```python
from build123d import *

# Parameters (mm, degrees)
SKETCH1_W           = 1025.461280364
SKETCH1_H           = 299.73488768
BOSS_EXTRUDE1_DEPTH = 19
SKETCH2_W           = 967.6
SKETCH2_H           = 175.74
CUT_EXTRUDE1_DEPTH  = 19
SKETCH3_R           = 7
CUT_EXTRUDE2_DEPTH  = 19
SKETCH5_W           = 19
SKETCH5_H           = 80
CUT_EXTRUDE3_DEPTH  = 19
SKETCH6_W           = 19
SKETCH6_H           = 80
CUT_EXTRUDE4_DEPTH  = 19


with BuildPart() as part:
    # Sketch1 → Boss-Extrude1 (new body)
    with BuildSketch(Plane.XY):
        with Locations((-1353.189241506, 613.368537441)):
            Rectangle(SKETCH1_W, SKETCH1_H)
    extrude(amount=BOSS_EXTRUDE1_DEPTH)

    # Sketch2 → Cut-Extrude1 (cut)
    with BuildSketch(Plane.XY.offset(19)):
        with Locations((-1352.119881688, 645.365981281)):
            Rectangle(SKETCH2_W, SKETCH2_H)
    extrude(amount=-CUT_EXTRUDE1_DEPTH, mode=Mode.SUBTRACT)

    # Sketch3 → Cut-Extrude2 (cut)
    with BuildSketch(Plane.XY.offset(19)):
        with Locations((-873.322364856, 728.339537454)):
            Circle(SKETCH3_R)
        with Locations((-873.322364856, 562.392425108)):
            Circle(SKETCH3_R)
    extrude(amount=-CUT_EXTRUDE2_DEPTH, mode=Mode.SUBTRACT)

    # Sketch5 → Cut-Extrude3 (cut)
    with BuildSketch(Plane(origin=(-840.458601324, 0, 0), x_dir=(0, 0, -1), z_dir=(1, 0, 0))):
        with Locations((-9.5, 643.235981281)):
            Rectangle(SKETCH5_W, SKETCH5_H)
    extrude(amount=-CUT_EXTRUDE3_DEPTH, mode=Mode.SUBTRACT)

    # Sketch6 → Cut-Extrude4 (cut)
    with BuildSketch(Plane.ZY.offset(1865.919881688)):
        with Locations((9.5, 643.235981281)):
            Rectangle(SKETCH6_W, SKETCH6_H)
    extrude(amount=-CUT_EXTRUDE4_DEPTH, mode=Mode.SUBTRACT)


solid = part.part
```
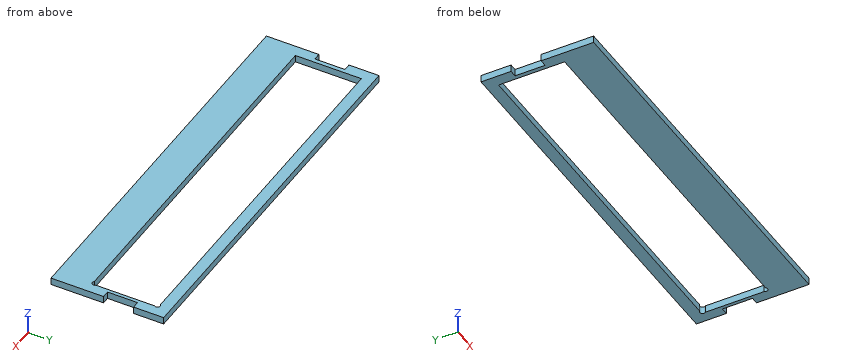
Could you check a few things on this model? Use its own coordinates, in mm. Coordinates: 2 decimals unless noted, no trailing zeros. Order: outer loops, then holes, each group sorted by start corner. A loop starts at its lowest first (then second) coordinate and runs counter-clockwise, first axis right, second up. Notation, with made-up numbers: M 73.25,-19 L 92.25,-19 A18 cw 92.25,-10 Z; hole C 3,50 d8. An arc over 180 degrees is marked long. Use one line per item in the form item = value. Start each with the question number.
1. Please list where these lines run through material, in increasing order: line 1 (Y direction, x = -994, z = 5.5); line 2 (X direction, y = 605, z = 16.25); line 3 (X direction, y = 593, z = 12).
2. Suppose I cut it at A-A on y = 693. Write out the boundary of the cut face in (x, z).
3. Suppose I cut it at C-C on z = 10.75. Write out the boundary of the cut face in (x, y), then the cut area to 3 significant figures.
4. Suppose I cut it at B-B on x = -1297.5. Write out the boundary of the cut face in (y, z).
Geometry says:
q1.line_1 = 463.5 to 557.5, 733.24 to 763.24
q1.line_2 = -1846.92 to -1835.92, -868.32 to -859.46
q1.line_3 = -1865.92 to -1835.92, -868.32 to -840.46
q2.outline = M -1865.92,0 L -1835.92,0 L -1835.92,19 L -1865.92,19 Z; M -868.32,0 L -840.46,0 L -840.46,19 L -868.32,19 Z
q3.outline = M -1865.92,463.5 L -840.46,463.5 L -840.46,603.24 L -859.46,603.24 L -859.46,683.24 L -840.46,683.24 L -840.46,763.24 L -1865.92,763.24 L -1865.92,683.24 L -1846.92,683.24 L -1846.92,603.24 L -1865.92,603.24 Z; hole M -1835.92,557.5 L -878.32,557.5 A7 ccw -868.32,567.29 L -868.32,723.44 A7 ccw -878.32,733.24 L -1835.92,733.24 Z
q3.area = 134,000 mm^2
q4.outline = M 463.5,0 L 557.5,0 L 557.5,19 L 463.5,19 Z; M 733.24,0 L 763.24,0 L 763.24,19 L 733.24,19 Z
